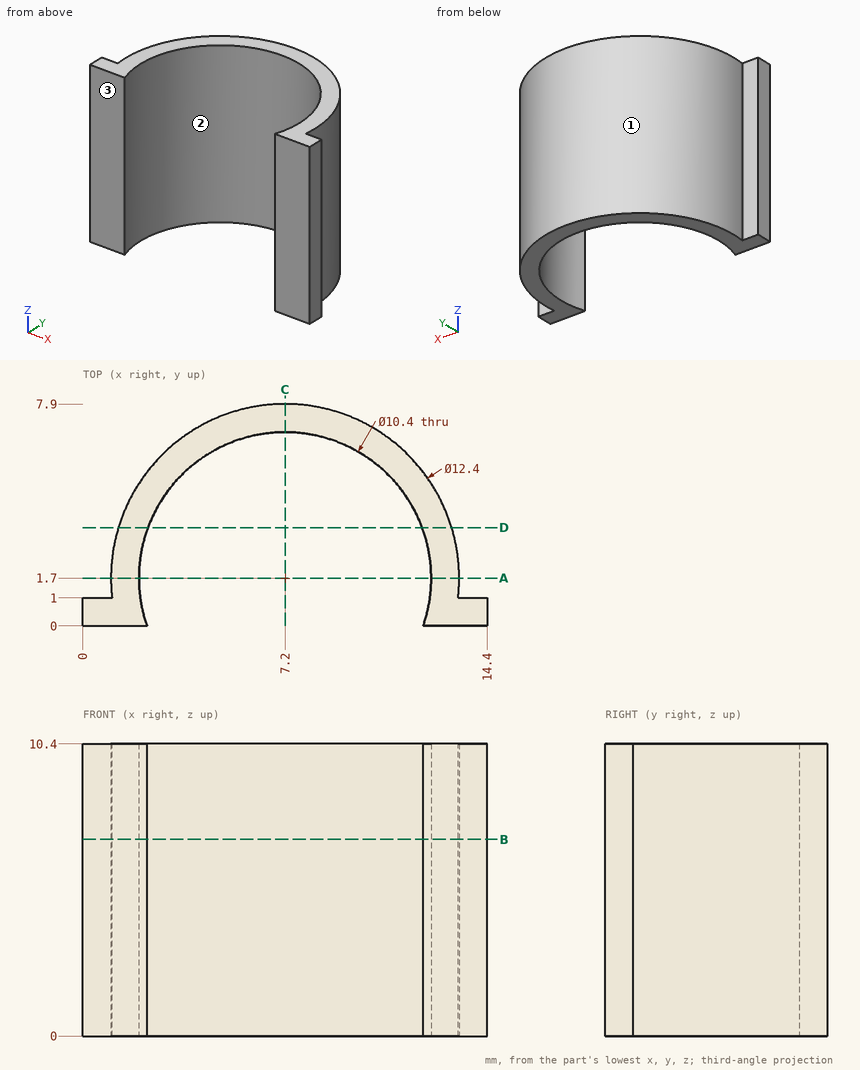
Can you work these out from the drawing? Everything is in mm from the part's minimum corner. Round coordinates to 2 decimals unless told otherwise and drop trailing zeros. Write each loop counter-clockwise with the first axis right and the second up, starting at its lowest first coordinate (ties: lowest second). Pieces come first, ordered by that corner, then holes. Notation, with made-up numbers: (-20, 36) - (15, 36) arc R13 cw to (15, 51) - close; hole circle Ø3 at (-39.75, 36). An arc over 180 degrees is marked (long way). Put each result on its own line as item: value. Start each with the question number.
(1) I want a section at C-C, the plane x = 7.2. Please give me the cut outline in (y, z), plus the area to 3 significant figures.
(2) Thinking about a two-plate mould opening in X: for the marked faces 1, 2 and 3, which applies, released by +X, released by -X, zero draft, split by the parting line, or undercut?
(3) I want a section at A-A, the plane y = 1.7. Please give me the cut outline in (x, z).
(4) I need wall thicknesses on probe 1 along X at (y, z) = (1.7, 3.25); probe 2 along Y at (x, z) = (7.2, 8.25); probe 3 along X at (y, z) = (4.5, 2.75). Which ranges of each line are inside material? Lowest first, please.
(5) Will these pins go through, and if not, where does the flat tip stop? pin 1 (1 mm diameter, centred on x = 9.5, z = 8.5, fed in from -Y); pin 2 (1.5 mm diameter, centred on x = 6, z = 5, fed in from -Y); pin 3 (0.5 mm diameter, centred on x = 14, z = 3.5, fed in from +Y).
(6) I want a section at D-D, the plane y = 3.5. Please give me the cut outline in (x, z).
(7) I want a section at B-B, the plane z = 7. Please give me the cut outline in (x, y), plus the area to 3 significant figures.
Here are the results:
1. outline: (6.9, 0) - (7.9, 0) - (7.9, 10.4) - (6.9, 10.4) - close
1. area: 10.4 mm^2
2. face 1: split by the parting line
2. face 2: undercut
2. face 3: zero draft
3. outline: (1, 0) - (2, 0) - (2, 10.4) - (1, 10.4) - close; (12.4, 0) - (13.4, 0) - (13.4, 10.4) - (12.4, 10.4) - close
4. probe 1: x = 1 to 2, 12.4 to 13.4
4. probe 2: y = 6.9 to 7.9
4. probe 3: x = 1.67 to 2.82, 11.58 to 12.73
5. pin 1: stops at y = 6.08
5. pin 2: stops at y = 6.52
5. pin 3: stops at y = 1
6. outline: (1.27, 0) - (2.32, 0) - (2.32, 10.4) - (1.27, 10.4) - close; (12.08, 0) - (13.13, 0) - (13.13, 10.4) - (12.08, 10.4) - close
7. outline: (0, 0) - (2.29, 0) arc R5.2 cw (long way) to (12.11, 0) - (14.4, 0) - (14.4, 1) - (13.36, 1) arc R6.2 ccw (long way) to (1.04, 1) - (0, 1) - close
7. area: 23.6 mm^2
